from build123d import *

# Parameters (mm, degrees)
SKETCH1_R           = 12.5
BOSS_EXTRUDE2_DEPTH = 50
CUT_REVOLVE1_ANGLE  = 270
CUT_EXTRUDE1_DEPTH  = 50


with BuildPart() as part:
    # Sketch1 → Boss-Extrude2 (new body)
    with BuildSketch(Plane.XY):
        with BuildLine():
            Line((0, 50), (50, 50))
            Line((50, 50), (50, 0))
            ThreePointArc((50, 0), (-35.355339059, -35.355339059), (0, 50))
        make_face()
        Circle(SKETCH1_R, mode=Mode.SUBTRACT)
    extrude(amount=BOSS_EXTRUDE2_DEPTH)

    # Sketch2 → Cut-Revolve1 (revolve, cut)
    with BuildSketch(Plane(origin=(0, 0, 0), x_dir=(0, 0, -1), z_dir=(1, 0, 0))):
        with BuildLine():
            Line((-41, 50), (-9, 50))
            ThreePointArc((-9, 50), (-25, 34), (-41, 50))
        make_face()
    revolve(axis=Axis((0, 0, 0), (0, 0, 1)), revolution_arc=CUT_REVOLVE1_ANGLE, mode=Mode.SUBTRACT)

    # Sketch2<2> → Cut-Extrude1 (cut)
    with BuildSketch(Plane(origin=(0, 0, 0), x_dir=(0, 0, -1), z_dir=(1, 0, 0))):
        with BuildLine():
            Line((-41, 50), (-9, 50))
            ThreePointArc((-9, 50), (-25, 34), (-41, 50))
        make_face()
    extrude(amount=CUT_EXTRUDE1_DEPTH, mode=Mode.SUBTRACT)


solid = part.part
Input: part model. Units: mm. Frame: model coordinates. A direction names the side the tool comes from. Give positions to 0.01 mm unless a question says otherwise; leave off trailing zeros. Order: outer loops, then holes, each group sorted by start corner. A loop starts at its lowest first (then second) coordinate and runs counter-clockwise, first axis right, second up. Notation, with made-up numbers: (14.25, 9.25) - (42.25, 9.25) arc R21 cw to (42.25, 22.25) - close; hole circle Ø2 at (-38.75, -23.75). An arc over 180 degrees is marked (long way). Answer as a JSON object with one key per item and string values. Group by question number.
Q1. Set-up query: faces 5 (the face through (44, 0, 25)), 6 (the face through (12, 12, 50)). Return all of +Z, -Z, +X, -X, +Y, -Y with unobstructed straight access to the full face (end or side cutting, diameter ignored); none if empty.
Q2. Mould query, pull axis Y, two halves, no side actions, for faces 1 (the face through (25, 50, 45)), 2 (the face through (-34.17, -36.5, 4.44)), 3 (the face through (12, 12, 0)), 4 (the face through (11.923, 3.755, 24.65)). Classes: pulls with the +Y half, pulls with the -Y half, needs draft (parallel to the pull), parting line crosses it, or undercut.
Q3. Cut plane A-A, the plane z = 25. Output: boundary loops of the cut face in (x, y).
Q4. Cut plane B-B, the plane z = 16.5. Output: boundary loops of the cut face in (x, y), then the cut area to 3 significant figures.
Q5. First-contact query: pin 1 Ø8 at (x, z) = (5, 25.5) entering from +Y; pin 2 Ø17.5 at (x, z) = (45.5, 26.5) entering from -Y; pin 3 Ø8 at (x, z) = (-3.5, 29.5) entering from +Y; pin 4 Ø2 at (x, y) = (36, 15.5) entering from -Z. Flat tips, straight axial feed; report the tip coordinate or a pass-through.
Q6. Line query: probe 1 along Y at (x, z) = (0, 39.5); probe 2 along Y at (x, z) = (0, 35); probe 3 along Z at (x, y) = (39, -16.5). Output: solid intervals per line, ascending.
Results:
{
 "1": {"face 5": "+X, -Y", "face 6": "+Z, +X, -X, +Y, -Y"},
 "2": {"face 1": "pulls with the +Y half", "face 2": "parting line crosses it", "face 3": "needs draft", "face 4": "undercut"},
 "3": {"outline": "(0, 34) arc R34 ccw (long way) to (34, 0) - (50, 0) - (50, 34) - close; hole circle Ø25 at (0, 0)"},
 "4": {"outline": "(0, 36.44) arc R36.44 ccw (long way) to (36.44, 0) - (50, 0) - (50, 36.44) - close; hole circle Ø25 at (0, 0)", "area": "4,460 mm^2"},
 "5": {"pin 1": "y = 34.65", "pin 2": "y = 0", "pin 3": "y = 36.3", "pin 4": "z = 0"},
 "6": {"probe 1": "-43.24 to -12.5, 12.5 to 43.24", "probe 2": "-37.51 to -12.5, 12.5 to 37.51", "probe 3": "0 to 10.95, 39.05 to 50"}
}
